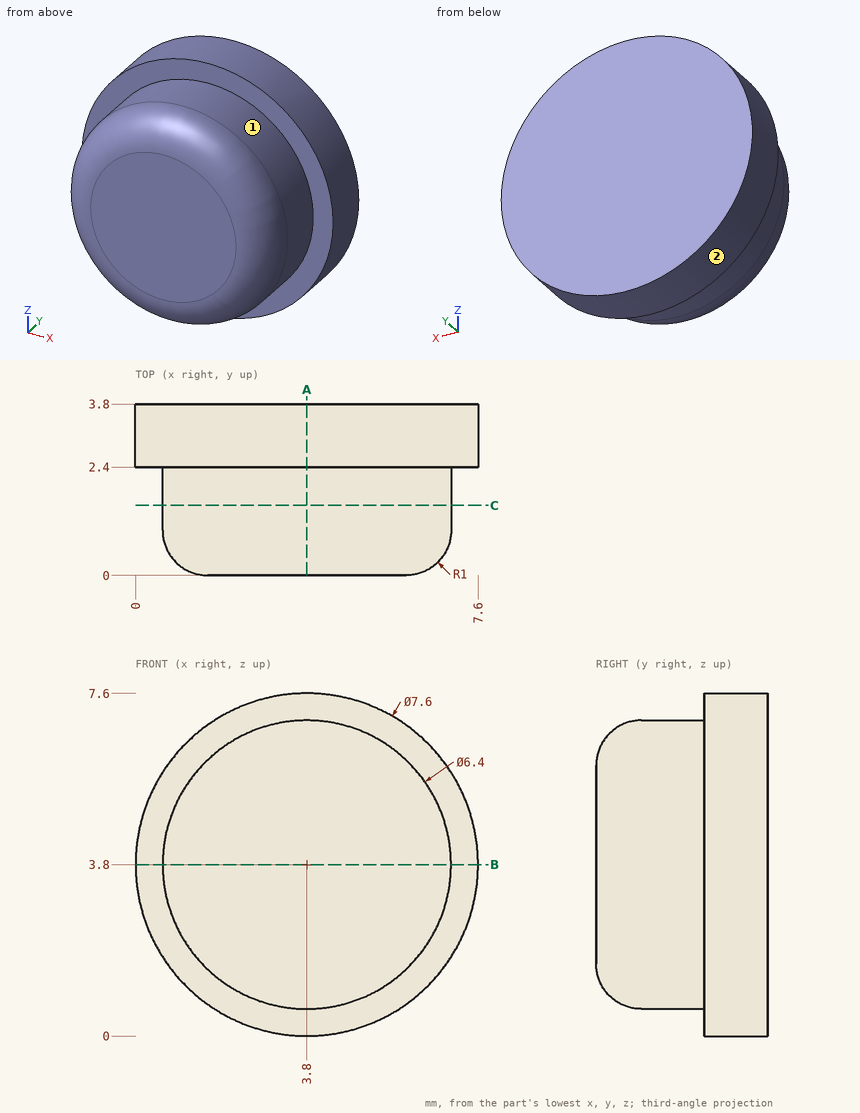
Design review of the part shown in the three views and the two pictorial views. Dimensions are in mm from the part's minimum x, y and z. A direction names the side the tool comes from. Round coordinates to 2 decimals unless told otherwise and drop trailing zeros. Loops run counter-clockwise (first coordinate to the right, second up) from the corner with the lowest first, then second, coordinate; pieces in that order, holes last.
Q1. To check wall thickness, follow line 1 along Y through (x, z) = (2, 0.75); line 2 along Y through (x, z) = (5.25, 6); line 3 along X through (y, z) = (0.6, 6.25). State the ranges of each line that lie inside material, in increasing order.
Result sheet:
line 1: y = 2.4 to 3.8
line 2: y = 0.1 to 3.8
line 3: x = 1.87 to 5.73
Q2. Add section A-A on x = 3.8. Write out the cut boundary in (y, z).
Result sheet:
outline: (0, 1.6) arc R1 ccw to (1, 0.6) - (2.4, 0.6) - (2.4, 0) - (3.8, 0) - (3.8, 7.6) - (2.4, 7.6) - (2.4, 7) - (1, 7) arc R1 ccw to (0, 6) - close
Q3. Machinability: for the marked faces 1 and 2, which of the approach directions +Z, -Z, +X, -X, +Y, -Y give a long, thin tool a straight path to every point of the face, cutting with its end or side? Answer none if there is none.
Result sheet:
face 1: -Y
face 2: +Y, -Y
Q4. Add section C-C on y = 1.55. Write out the cut boundary in (x, z), plus the area to 3 significant figures.
Result sheet:
outline: circle Ø6.4 at (3.8, 3.8)
area: 32.2 mm2
Q5. Insertion check: pin 1 Ø1 at (y, z) = (2.5, 1) entering from +X; pin 2 Ø2 at (y, z) = (3.5, 5.5) entering from -X. Each pin has a flat end and moves straight along its axis. Give the tip position at first contact, or say it passes through.
Result sheet:
pin 1: stops at x = 6.82
pin 2: stops at x = 0.07
Q6. Add section B-B on z = 3.8. Write out the cut boundary in (x, y), plus the area to 3 significant figures.
Result sheet:
outline: (0, 2.4) - (0.6, 2.4) - (0.6, 1) arc R1 ccw to (1.6, 0) - (6, 0) arc R1 ccw to (7, 1) - (7, 2.4) - (7.6, 2.4) - (7.6, 3.8) - (0, 3.8) - close
area: 25.6 mm2
